Answer from the drawing. Dimensions are ordinates in mm from the lowest x, y and z of the part. Coordinates: 2 decimals unless noted, no trailing zeros. Write each loop counter-clockwise with the first axis right and the second up, starting at its lowest first coordinate (ties: lowest second). Pieces come first, ordered by that corner, then holes.
(1) Find the intervals of material crossed by probe 1 along Z at (x, y) = (875, 11.5); probe 2 along X at (y, z) = (7.75, 175); probe 3 along X at (y, z) = (2, 26), in increasing order.
(2) Section B-B on y = 8 is taken. Write down the section's boundary in (x, z).
(3) Section A-A on x = 759 is taken. Write down the section's boundary in (y, z), then the cut area to 3 significant figures.
(4) Given pin 1 (13 mm diameter, centred on x = 25, z = 25, fed in from +Y); pin 2 (6 mm diameter, centred on x = 25, z = 175, fed in from -Y), each flat-ended and moving along its own axis, determine where each tip first touches the part or whether it passes through.
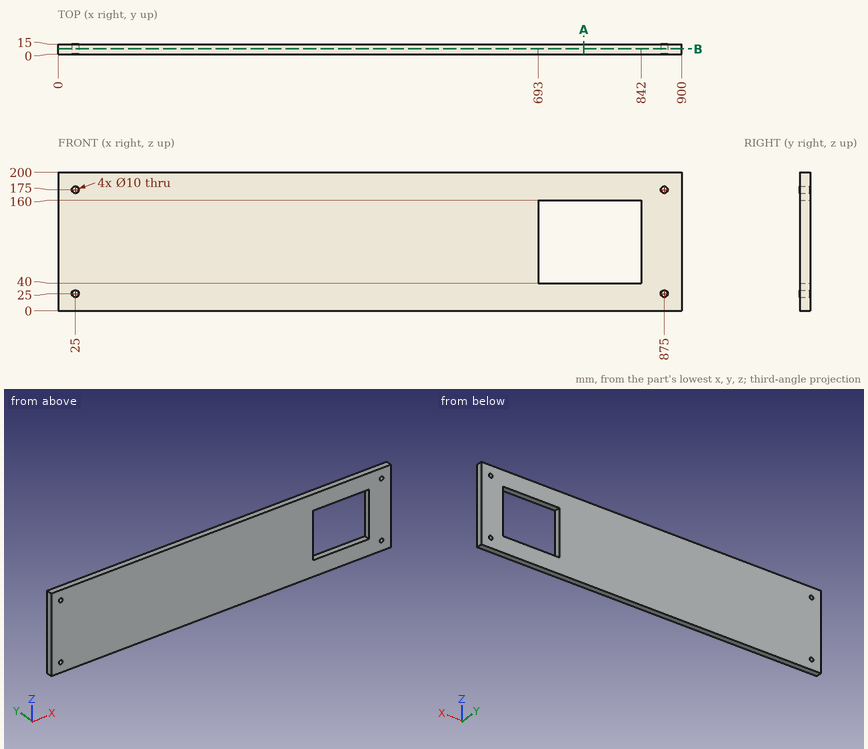
Response:
1. probe 1: z = 0 to 20, 30 to 170, 180 to 200
1. probe 2: x = 0 to 20, 30 to 870, 880 to 900
1. probe 3: x = 0 to 20.1, 29.9 to 870.1, 879.9 to 900
2. outline: (0, 0) - (900, 0) - (900, 200) - (0, 200) - close; hole circle Ø10 at (25, 25); hole circle Ø10 at (25, 175); hole (693, 40) - (842, 40) - (842, 160) - (693, 160) - close; hole circle Ø10 at (875, 25); hole circle Ø10 at (875, 175)
3. outline: (0, 0) - (15, 0) - (15, 40) - (0, 40) - close; (0, 160) - (15, 160) - (15, 200) - (0, 200) - close
3. area: 1,200 mm2
4. pin 1: stops at y = 15
4. pin 2: passes through
